Autodesk Inventor part; units mm, degrees
ref_plane "YZ Plane" through (0, 0, 0) normal (1, 0, 0) x (0, 1, 0)
ref_plane "XZ Plane" through (0, 0, 0) normal (0, 1, 0) x (-1, 0, 0)
ref_plane "XY Plane" through (0, 0, 0) normal (0, 0, 1) x (1, 0, 0)
sketch "Skizze1" plane through (0, 0, 0) normal (0, 0, 1) x (1, 0, 0)
  line L0 (-41.9152, 0) -> (-41.9152, -12)
  line L1 (-53.9134, -12) -> (-41.9152, -12)
  line L2 (-53.9134, 0) -> (-53.9134, -12)
  line L3 (-41.9152, 0) -> (-53.9134, 0)
  line L4 (-39.4739, 0) -> (-39.4739, -12)
  line L5 (-41.9558, -12.0406) -> (-53.9549, -0.0415) construction
  line L6 (-53.9549, -11.9585) -> (-41.9558, 0.0406) construction
  circle A0 centre (-47.9553, -5.959) radius 1.675
  line L7 (-39.4739, -12) -> (-53.9134, -12)
  line L8 (-53.9134, -12) -> (-53.9134, 0)
  line L9 (-53.9134, 0) -> (-39.4739, 0)
  line L10 (-39.4739, 0) -> (-39.4739, -12)
  point P0 (0, 0)
  point P1 (-39.4739, 0)
  dimension "d0" = 3.35
extrude "Extrusion1" add sketch "Skizze1" along normal blind 6.4 contours L9 L4 L7 L0 | L0 L1 L2 L3 | A0
sketch "Skizze2" plane through (0, 0, 0) normal (0, 0, -1) x (-1, 0, 0)
  circle A0 centre (47.9553, -5.959) radius 1.675
  point P0 (0, 0)
extrude "Extrusion2" cut sketch "Skizze2" against normal blind 5.4
chamfer "Fase1" distance 0.6 angle 45 1 edges at (-46.2803, -5.959, 0)
properties part number "13_Motor_Fixation_Thread_Mount"
For this review, take the finished solid that the model builds, in its own axes (mm). Coordinates: 2 decimals unless noted, no trailing zeros. Loops run counter-clockwise (first coordinate to the right, second up) from the corner with the lowest first, then second, coordinate; pieces in that order, holes last. Notation, with made-up numbers: (12.5, 54) -> (51.5, 54) arc R19 ccw to (51.5, 74) -> close; hole circle Ø1 at (-2, 14.5). An arc over 180 degrees is marked (long way). Write each question's results on one line, items separated by ' | '.
Q1. For pin 1 Ø2 at (x, z) = (-49.5, 4.5) entering from +Y; pin 2 Ø2.5 at (x, y) = (-48, -5) entering from -Z, all flat-tipped, find the tip position at first contact; note any pin that passes through.
Taken from the geometry:
pin 1: y = 0 | pin 2: z = 0.06
Q2. Mouldability with a two-part tool opening along Y and no side actions: class faces 1 (the flat face through (-47, -12, 3)), 2 (the flat face through (-48, -6, 5.4)), 3 (the cylindrical face through (-49.503, -6.601, 2.966)), 4 (the flat face through (-47, -6, 6.4)) as +Y half, -Y half, draft (parallel to the pull), parting line (faces both ways), or undercut.
Taken from the geometry:
face 1: -Y half | face 2: undercut | face 3: undercut | face 4: draft
Q3. To check wall thickness, follow line 1 along Y through (x, z) = (-48, 3); line 2 along X through (y, z) = (-6.75, 3); line 3 along X through (y, z) = (-7, 1.25). State the ranges of each line that lie inside material, in increasing order. Write a range as [from, to].
Taken from the geometry:
line 1: [-12, -7.63], [-4.28, 0] | line 2: [-53.91, -49.43], [-46.48, -39.47] | line 3: [-53.91, -49.27], [-46.64, -39.47]
Q4. Add section A-A, the plane z = 4.25. State the section outline as (x, y) points (3 decimals).
Taken from the geometry:
outline: (-53.913, -12) -> (-39.474, -12) -> (-39.474, 0) -> (-53.913, 0) -> close; hole circle Ø3.35 at (-47.955, -5.959)
